```python
from build123d import *

# Parameters (mm, degrees)
F0_W     = 101.6
F0_H     = 101.6
F1_DEPTH = 101.6
F2_R     = 25.4
F3_DEPTH = 101.6
F6_W     = 50.8
F6_H     = 50.8
F7_DEPTH = 101.6
F8_R     = 6.35


with BuildPart() as f1:
    # F0 (on Top) → F1 (new body)
    with BuildSketch(Plane.XY):
        Rectangle(F0_W, F0_H)
    extrude(amount=F1_DEPTH)

    # F2 (on face) → F3 (join)
    with BuildSketch(Plane.XY.offset(101.6)):
        Circle(F2_R)
    extrude(amount=F3_DEPTH)

    # F4 (on face) → F5 (revolve)
    with BuildSketch(Plane.XY.offset(203.2)):
        with BuildLine():
            Line((0, -25.4), (0, -38.1))
            ThreePointArc((0, -38.1), (38.1, 0), (0, 38.1))
            Line((0, 38.1), (0, 25.4))
            ThreePointArc((0, 25.4), (17.960512, 17.960512), (25.4, 0))
            ThreePointArc((25.4, 0), (17.960512, -17.960512), (0, -25.4))
        make_face()
        with BuildLine():
            ThreePointArc((0, 25.4), (-25.4, 0), (0, -25.4))
            Line((0, -25.4), (0, 0))
            Line((0, 0), (0, 25.4))
        make_face()
    revolve(axis=Axis((0, -19.05, 203.2), (0, 1, 0)))

    # F6 (on face) → F7 (cut)
    with BuildSketch(Plane.XZ.offset(50.8)):
        with Locations((0, 50.8)):
            Rectangle(F6_W, F6_H)
    extrude(amount=-F7_DEPTH, mode=Mode.SUBTRACT)

    # F8
    f8_edges = [f1.edges().sort_by_distance(p)[0] for p in [
        (-50.8, 0, 101.6),
        (0, -50.8, 101.6),
        (50.8, 0, 101.6),
        (0, 50.8, 101.6),
        (50.8, 50.8, 50.8),
        (50.8, -50.8, 50.8),
        (50.8, 0, 0),
        (0, -50.8, 0),
        (-50.8, -50.8, 50.8),
        (-50.8, 50.8, 50.8),
        (-50.8, 0, 0),
        (-25.4, 0, 101.6),
        (25.4, 0, 138.200968),
        (-25.4, 0, 174.801937),
    ]]
    fillet(f8_edges, radius=F8_R)


solid = f1.part
```
The listing builds one solid part. Answer for the finished solid, in the listing's coordinates (mm). A direction names the side the tool comes from. Give positions to 0.01 mm unless a question says otherwise; leave off trailing zeros. Order: outer loops, then holes, each group sorted by start corner. A loop starts at its lowest first (then second) coordinate and runs counter-clockwise, first axis right, second up. Notation, with made-up numbers: (66.5, -21.75) -> (117.5, -21.75) arc R31 cw to (117.5, 8.25) -> close; hole circle Ø10 at (6, -13). An arc over 180 degrees is marked (long way). One line per item, written item: value.
1) Find section B-B, the plane z = 117. Determine the outline of the cut face in (x, y), plus the area to 3 significant figures.
Reported:
outline: circle Ø50.8 at (0, 0)
area: 2,030 mm^2
2) Determine the mould class of faces 4 (the flat face through (-50.8, -1, 50)), 5 (the cylindrical face through (48.89, 48.99, 48.29)), 6 (the cylindrical face through (0.62, 48.89, 99.79)), 7 (the flat face through (25.4, -1, 50)) for opening direction X: pulls with the +X half, pulls with the -X half, needs draft (parallel to the pull), parting line crosses it, or undercut.
Reported:
face 4: pulls with the -X half
face 5: pulls with the +X half
face 6: needs draft
face 7: undercut
3) Find the intervals of material crossed by line 1 (X direction, y = -41, z = 29.5); line 2 (Z direction, x = -12.5, y = 30); line 3 (Z direction, x = -22.5, y = -43), in increasing order.
Reported:
line 1: x = -50.8 to -25.4, 25.4 to 50.8
line 2: z = 0 to 25.4, 76.2 to 101.6, 183.32 to 223.08
line 3: z = 0 to 25.4, 76.2 to 101.6
4) A tool of negligible diameter and unlimited length cuts with its end or side. For faces 1 (the cylindrical face through (0.62, -48.89, 99.79)), 2 (the flat face through (0, -1, 76.2)), 3 (the flat face through (-11, 30, 101.6)), from which of +Z, -Z, +X, -X, +Y, -Y can it reach the whole face along a straight path? Write none if from no direction.
Reported:
face 1: +Z, +X, -X, -Y
face 2: +Y, -Y
face 3: none
5) Flat-ended cylindrical pins translate along their axes: P1, Ø5, axis at x = -14.5, z = 158.5, coming from the +Y side; P2, Ø3, axis at x = 25, y = -7, coming from the +Z side; P3, Ø1, axis at x = 34.5, y = 5, coming from the +Z side. Find the tip coordinate at first contact, or state that the pin passes through.
Reported:
P1: stops at y = 22.39
P2: stops at z = 232.41
P3: stops at z = 219.66
6) Find section A-A, the plane y = 41.5. Determine the outline of the cut face in (x, z), plus the area to 3 significant figures.
Reported:
outline: (-50.8, 6.35) arc R6.35 ccw to (-44.45, 0) -> (44.45, 0) arc R6.35 ccw to (50.8, 6.35) -> (50.8, 95.25) arc R6.35 ccw to (44.45, 101.6) -> (-44.45, 101.6) arc R6.35 ccw to (-50.8, 95.25) -> close; hole (-25.4, 25.4) -> (25.4, 25.4) -> (25.4, 76.2) -> (-25.4, 76.2) -> close
area: 7,710 mm^2
